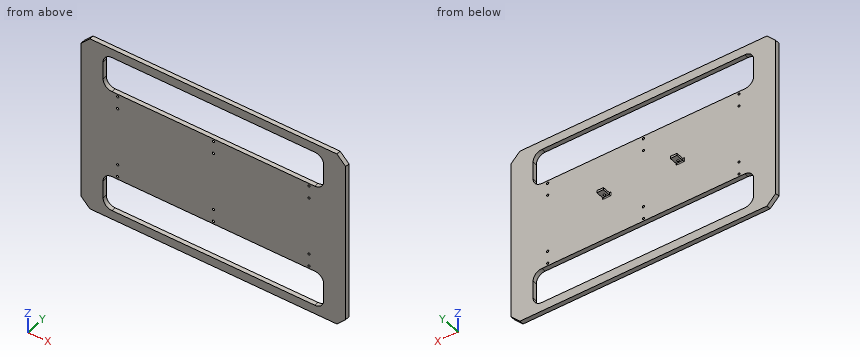
from build123d import *

# Parameters (mm, degrees)
BOSS_EXTRUDE1_DEPTH           = 5
CUT_EXTRUDE1_DEPTH            = 361.589794642
CUT_EXTRUDE1_DEPTH_BACK       = 361.589794642
SKETCH3_W                     = 7.5
SKETCH3_H                     = 5
BOSS_EXTRUDE2_DEPTH           = 20
F_5_0MM_START                 = -2.5
F_5_0MM_DOWEL_HOLE1_OUTLINE_R = 2.5
F_5_0MM_DOWEL_HOLE1_DEPTH     = 5
FILLET1_R                     = 2
F_5_0MM_DOWEL_HOLE3_D         = 5


# Read off the part's stored shape, not the designer's step: Ø5.0mm Dowel Hole1
with BuildPart() as part:
    # Sketch1 → Boss-Extrude1 (new, symmetric)
    with BuildSketch(Plane(origin=(0, 0, 0), x_dir=(1, 0, 0), z_dir=(0, 1, 0))):
        Polygon((-300, 180), (-280, 200), (280, 200), (300, 180), (300, -180), (280, -200), (-280, -200), (-300, -180), align=None)
    extrude(amount=BOSS_EXTRUDE1_DEPTH, both=True)

    # Sketch2 → Cut-Extrude1 (cut, two sides: drawn at the far end of the back side and taken through both)
    with BuildSketch(Plane(origin=(0, 0, 0), x_dir=(1, 0, 0), z_dir=(0, 1, 0)).offset(-CUT_EXTRUDE1_DEPTH_BACK)):
        with BuildLine():
            Line((-230, 180), (230, 180))
            ThreePointArc((230, 180), (244.142135624, 174.142135624), (250, 160))
            Line((250, 160), (250, 120))
            ThreePointArc((250, 120), (244.142135624, 105.857864376), (230, 100))
            Line((230, 100), (-230, 100))
            ThreePointArc((-230, 100), (-244.142135624, 105.857864376), (-250, 120))
            Line((-250, 120), (-250, 160))
            ThreePointArc((-250, 160), (-244.142135624, 174.142135624), (-230, 180))
        make_face()
        with BuildLine():
            Line((250, -160), (250, -120))
            ThreePointArc((250, -120), (244.142135624, -105.857864376), (230, -100))
            Line((230, -100), (-230, -100))
            ThreePointArc((-230, -100), (-244.142135624, -105.857864376), (-250, -120))
            Line((-250, -120), (-250, -160))
            ThreePointArc((-250, -160), (-244.142135624, -174.142135624), (-230, -180))
            Line((-230, -180), (230, -180))
            ThreePointArc((230, -180), (244.142135624, -174.142135624), (250, -160))
        make_face()
    extrude(amount=CUT_EXTRUDE1_DEPTH + CUT_EXTRUDE1_DEPTH_BACK, mode=Mode.SUBTRACT)

    # Sketch3 → Boss-Extrude2 (add)
    with BuildSketch(Plane(origin=(0, 5, 0), x_dir=(1, 0, 0), z_dir=(0, 1, 0))):
        with Locations((-87.083333333, 0)):
            Rectangle(SKETCH3_W, SKETCH3_H)
        with Locations((-79.583333333, 0)):
            Rectangle(SKETCH3_W, SKETCH3_H)
        with Locations((79.583333333, 0)):
            Rectangle(SKETCH3_W, SKETCH3_H)
        with Locations((87.083333333, 0)):
            Rectangle(SKETCH3_W, SKETCH3_H)
    extrude(amount=BOSS_EXTRUDE2_DEPTH)

    # Ø5.0mm Dowel Hole1 outline → Ø5.0mm Dowel Hole1 (cut)
    with BuildSketch(Plane.XY.offset(F_5_0MM_START)):
        with Locations((83.333333333, 11.67)):
            Circle(F_5_0MM_DOWEL_HOLE1_OUTLINE_R)
        with Locations((-83.333333333, 11.67)):
            Circle(F_5_0MM_DOWEL_HOLE1_OUTLINE_R)
    extrude(amount=F_5_0MM_DOWEL_HOLE1_DEPTH, mode=Mode.SUBTRACT)

    # Fillet1
    fillet1_edges = [part.edges().sort_by_distance(p)[0] for p in [
        (-90.833333333, 5, 0),
        (-83.333333333, 5, 2.5),
        (-83.333333333, 5, -2.5),
        (-75.833333333, 5, 0),
        (75.833333333, 5, 0),
        (83.333333333, 5, 2.5),
        (83.333333333, 5, -2.5),
        (90.833333333, 5, 0),
    ]]
    fillet(fillet1_edges, radius=FILLET1_R)

    # Ø5.0mm Dowel Hole3 (through all)
    with Locations(Plane(origin=(0, 5, 0), x_dir=(1, 0, 0), z_dir=(0, 1, 0))):
        with Locations((-217, 94), (-217, 66), (-217, -94), (-217, -66), (0, 94), (0, 66), (0, -66), (0, -94), (217, -94), (217, -66), (217, 66), (217, 94)):
            Hole(F_5_0MM_DOWEL_HOLE3_D / 2)


solid = part.part
For this review, take the finished solid that the model builds, in its own axes (mm). Round coordinates to 2 decimals unless told otherwise and drop trailing zeros. Order: outer loops, then holes, each group sorted by start corner. A loop starts at its lowest first (then second) coordinate and runs counter-clockwise, first axis right, second up. Notation, with made-up numbers: M -3,-11 L 49,-11 A7 ccw 49,-1 Z; hole C 23,28 d8. An arc over 180 degrees is marked long. Write each question's results on one line, items separated by ' | '. Start each with the question number.
1. Add section C-C (x = -261.5). State the section outline as (y, z) points.
2. Add section B-B (y = 18.75). State the section outline as (x, z) points, then the cut area to 3 significant figures.
3. Add section A-A (x = 186). State the section outline as (y, z) points.
4. To check wall thickness, follow L1, parallel to X at y = 2, z = 66; L2, parallel to Z at x = 36.5, y = 3.5; L3, parallel to Y at x = -43.5, z = -38.5. State the ranges of each line that lie inside material, in increasing order. Write a range as [from, to].
5. Clearance check with flat-ended pins moving along their axes: pin 1 Ø4.5 at (x, y) = (80, 15) entering from +Z; pin 2 Ø5.5 at (y, z) = (13, -0.5) entering from +X; pin 3 Ø3 at (x, z) = (217, 94) entering from -Y; pin 4 Ø7.5 at (x, y) = (84, 19) entering from -Z. State where each tip first meets the part, or that it passes through.
Output values:
1) outline: M -5,-200 L 5,-200 L 5,200 L -5,200 Z
2) outline: M -90.83,-2.5 L -75.83,-2.5 L -75.83,2.5 L -90.83,2.5 Z; M 75.83,-2.5 L 90.83,-2.5 L 90.83,2.5 L 75.83,2.5 Z | area: 150 mm^2
3) outline: M -5,-200 L 5,-200 L 5,-180 L -5,-180 Z; M -5,-100 L 5,-100 L 5,100 L -5,100 Z; M -5,180 L 5,180 L 5,200 L -5,200 Z
4) L1: [-300, -219.5], [-214.5, -2.5], [2.5, 214.5], [219.5, 300] | L2: [-200, -180], [-100, 100], [180, 200] | L3: [-5, 5]
5) pin 1: z = 2.5 | pin 2: x = 90.83 | pin 3: through | pin 4: z = -2.5
